Design review of the part built by this model. Coordinates are the model's own, in mm. A direction names the side the tool comes from. Coordinates: 2 decimals unless noted, no trailing zeros. Write each loop counter-clockwise with the first axis right and the second up, starting at its lowest first coordinate (ties: lowest second). Pieces come first, ordered by that corner, then holes. Notation, with made-up numbers: (83, 19) - (109, 19) arc R15 ccw to (109, 29) - close; hole circle Ø1 at (7, 31.5). An arc over 180 degrees is marked (long way). Answer as a JSON object with one key per item and string values.
```python
from build123d import *

# Parameters (mm, degrees)
SKETCH_1_W          = 43
SKETCH_1_H          = 33.5
EXTRUDE_1_DEPTH     = 3
EXTRUDE_1_DRAFT     = 15
SKETCH_2_W          = 43
SKETCH_2_H          = 33
EXTRUDE_2_DEPTH     = 5
SKETCH_3_W          = 20
SKETCH_3_H          = 7
CUT_EXTRUDE_1_DEPTH = 39
SKETCH_4_W          = 8
SKETCH_4_H          = 18
CUT_EXTRUDE_2_DEPTH = 1
CHAMFER_1_SIZE      = 1
CHAMFER_2_SIZE      = 6
CHAMFER_3_SIZE      = 4
SKETCH_5_W          = 20
SKETCH_5_H          = 3
CUT_EXTRUDE_3_DEPTH = 48.454342555


with BuildPart() as part:
    # Эскиз1 → Бобышка-Вытянуть1 (with draft: the straight prism first)
    with BuildSketch(Plane(origin=(0, 0, 0), x_dir=(1, 0, 0), z_dir=(0, 1, 0))):
        Rectangle(SKETCH_1_W, SKETCH_1_H)
    extrude(amount=-EXTRUDE_1_DEPTH)
    # Бобышка-Вытянуть1: the draft: its side faces are tilted about the plane it starts from
    extrude_1_sides = [part.faces().sort_by_distance(p)[0] for p in [
        (21.5, -1.5, 0),
        (0, -1.5, -16.75),
        (-21.5, -1.5, 0),
        (0, -1.5, 16.75),
    ]]
    draft(extrude_1_sides, Plane(origin=(0, 0, 0), x_dir=(1, 0, 0), z_dir=(0, 1, 0)), EXTRUDE_1_DRAFT)

    # Эскиз2 → Бобышка-Вытянуть2 (add)
    with BuildSketch(Plane(origin=(0, 0, 0), x_dir=(1, 0, 0), z_dir=(0, 1, 0))):
        Rectangle(SKETCH_2_W, SKETCH_2_H)
    extrude(amount=EXTRUDE_2_DEPTH)

    # Эскиз3 → Вырез-Вытянуть1 (cut)
    with BuildSketch(Plane(origin=(21.5, 0, 0), x_dir=(0, 0, -1), z_dir=(1, 0, 0))):
        Rectangle(SKETCH_3_W, SKETCH_3_H)
    extrude(amount=-CUT_EXTRUDE_1_DEPTH, mode=Mode.SUBTRACT)

    # Эскиз4 → Вырез-Вытянуть2 (cut)
    with BuildSketch(Plane.XZ.offset(-3.5)):
        with Locations((14.5, 0)):
            Rectangle(SKETCH_4_W, SKETCH_4_H)
    extrude(amount=-CUT_EXTRUDE_2_DEPTH, mode=Mode.SUBTRACT)

    # Фаска1
    chamfer_1_edges = [part.edges().sort_by_distance(p)[0] for p in [
        (21.5, 3.5, 0),
    ]]
    chamfer(chamfer_1_edges, length=CHAMFER_1_SIZE)

    # Фаска2
    # the kernel refuses this chamfer: 6 mm, written as the material it takes off along each edge
    with BuildSketch(Plane(origin=(-17.5, -3, -10), x_dir=(0.027495876610586202, 0.9996219169112968, 0), z_dir=(0, 0, 1))) as chamfer_2_piece_1:
        Polygon((CHAMFER_2_SIZE * 0.999621916911, CHAMFER_2_SIZE * 0.0274958766106), (-CHAMFER_2_SIZE * 0.0274958766106, CHAMFER_2_SIZE * 0.999621916911), (0, 0), align=None)
    extrude(amount=20, mode=Mode.SUBTRACT)

    # Фаска3
    chamfer_3_edges = [part.edges().sort_by_distance(p)[0] for p in [
        (0, 5, -16.5),
        (0, 5, 16.5),
    ]]
    chamfer(chamfer_3_edges, length=CHAMFER_3_SIZE)

    # Эскиз5 → Вырез-Вытянуть3 (cut, through all)
    with BuildSketch(Plane.ZY.offset(-21.5)):
        with Locations((0, -1.5)):
            Rectangle(SKETCH_5_W, SKETCH_5_H)
    extrude(amount=-CUT_EXTRUDE_3_DEPTH, mode=Mode.SUBTRACT)


solid = part.part
```
(1) Tool access review of faces 4 (the face through (21.5, 4.7, 0.2)), 5 (the face through (-0.3, 0.5, 16.5)), 6 (the face through (14, 4, 9)), 7 (the face through (-0.3, 0.5, -16.5)): name each direction out of +Z, -Z, +X, -X, +Y, -Y from which nothing blocks a thin tool from reaching the whole face with its end or side.
Solved:
{"face 4": "+Z, -Z, +X, +Y", "face 5": "+Z, +X, -X, +Y", "face 6": "-Y", "face 7": "-Z, +X, -X, +Y"}
(2) Take a section at C-C, the plane z = 13. Write out the cut boundary in (x, y), and give its area (3 significant figures).
Solved:
{"outline": "(-22.3, -3) - (22.3, -3) - (21.5, 0) - (21.5, 4.5) - (-21.5, 4.5) - (-21.5, 0) - close", "area": "325 mm^2"}
(3) For pin 1 (6 mm diameter, centred on x = 9.5, z = -4.5, fed in from -Y); pin 2 (3 mm diameter, centred on y = 3.5, z = -6.5, fed in from +X); pin 3 (1.1 mm diameter, centred on x = 13, y = 4, fed in from -Z), all flat-tipped, find the tip position at first contact; note any pin that passes through.
Solved:
{"pin 1": "stops at y = 3.5", "pin 2": "stops at x = 21.5", "pin 3": "stops at z = -14.05"}
(4) Take a section at B-B, the plane x = 11. Write out the cut boundary in (y, z).
Solved:
{"outline": "(-3, -17.55) - (0, -16.75) - (0, -16.5) - (1, -16.5) - (5, -12.5) - (5, 12.5) - (1, 16.5) - (0, 16.5) - (0, 16.75) - (-3, 17.55) - (-3, 10) - (3.5, 10) - (3.5, 9) - (4.5, 9) - (4.5, -9) - (3.5, -9) - (3.5, -10) - (-3, -10) - close"}
(5) Take a section at A-A, the plane y = 1.5. Write out the cut boundary in (x, z).
Solved:
{"outline": "(-21.5, -16) - (21.5, -16) - (21.5, -10) - (-19, -10) - (-19, 10) - (21.5, 10) - (21.5, 16) - (-21.5, 16) - close"}
(6) Take a section at D-D, the plane z = 5. Write out the cut boundary in (x, y).
Solved:
{"outline": "(-21.87, -1.37) - (-17.5, 3) - (-17.5, 3.5) - (10.5, 3.5) - (10.5, 4.5) - (18.5, 4.5) - (18.5, 3.5) - (20.5, 3.5) - (21.5, 4.5) - (21.5, 5) - (-21.5, 5) - (-21.5, 0) - close"}
(7) The part is to be moulded in two halves that separate along X. For faces 1 (the face through (-0.312, -1.479, 17.146)), 2 (the face through (-19.7, 0.8, -0.1)), 3 (the face through (18.5, 4, 0)), say which applies: pulls with the +X half, pulls with the -X half, needs draft (parallel to the pull), parting line crosses it, or undercut.
Solved:
{"face 1": "needs draft", "face 2": "pulls with the +X half", "face 3": "undercut"}
(8) To check wall thickness, follow line 1 (Z direction, x = -8, y = -2); line 2 (Z direction, x = 14, y = -0.5); line 3 (X direction, y = 0.75, z = -12). State the ranges of each line that lie inside material, in increasing order. Write a range as from..to.
Solved:
{"line 1": "z = -17.29..-10, 10..17.29", "line 2": "z = -16.88..-10, 10..16.88", "line 3": "x = -21.5..21.5"}
